Source: CAD feature listing. Evaluate the final solid. Frame: model axes, mm. A direction names the side the tool comes from. Give positions to 0.01 mm unless a question says otherwise; leave off trailing zeros. Order: outer loops, then holes, each group sorted by start corner. A loop starts at its lowest first (then second) coordinate and runs counter-clockwise, first axis right, second up. Notation, with made-up numbers: M 41.25,56 L 74.25,56 A32 cw 74.25,82 Z; hole C 67,-28.5 d9. An arc over 180 degrees is marked long. Return JSON: item names as keys, results as strings.
Autodesk Inventor part; units mm, degrees
ref_plane "YZ Plane" through (0, 0, 0) normal (1, 0, 0) x (0, 1, 0)
ref_plane "XZ Plane" through (0, 0, 0) normal (0, 1, 0) x (-1, 0, 0)
ref_plane "XY Plane" through (0, 0, 0) normal (0, 0, 1) x (1, 0, 0)
sketch "Sketch1" plane through (0, 0, 0) normal (0, 0, 1) x (1, 0, 0)
  line L0 (-84.0821, 192.7052) -> (642.9929, 192.7052)
  line L1 (642.9929, 192.7052) -> (642.9929, -137.4948)
  line L2 (642.9929, -137.4948) -> (-84.0821, -137.4948)
  line L3 (-84.0821, -137.4948) -> (-84.0821, 192.7052)
  circle A0 centre (131.8179, -91.7748) radius 25.4
  circle A1 centre (318.0537, 116.5052) radius 12.7
  line L4 (642.9929, -137.4948) -> (592.1929, -137.4948)
  line L5 (592.1929, -137.4948) -> (592.1929, -73.9948)
  line L6 (592.1929, -73.9948) -> (642.9929, -73.9948)
  line L7 (642.9929, -73.9948) -> (642.9929, -137.4948)
  line L8 (642.9929, 192.7052) -> (592.6352, 192.7052)
  line L9 (642.9929, 2.2052) -> (642.9929, 192.7052)
  line L10 (-84.0821, 53.0052) -> (5.7204, 53.0052) construction
  line L11 (-84.0821, 65.7052) -> (68.3179, -137.4948)
  line L12 (595.3679, 192.7052) -> (595.3679, 2.2052)
  line L13 (595.3679, 2.2052) -> (642.9929, 2.2052)
  point P0 (0, 0)
  dimension "d0" = 727.075
  dimension "d2" = 50.8
  dimension "d3" = 25.4
  dimension "d4" = 215.9
  dimension "d5" = 279.4
  dimension "d14" = 152.4
  dimension "d15" = 203.2
  dimension "d16" = 330.2
  dimension "d17" = 63.5
  dimension "d19" = 50.8
  dimension "d20" = 139.7
  dimension "d21" = 45.72
  dimension "d22" = 254
extrude "Extrusion1" add sketch "Sketch1" along normal blind 9.525 contours L0 L12 L13 L1 L6 L5 L2 L11 L3
sketch "Sketch3" plane through (0, 0, 9.525) normal (0, 0, 1) x (1, 0, 0)
  line L0 (595.3679, 2.2052) -> (595.3679, 192.7052)
  line L1 (595.3679, 192.7052) -> (-84.0821, 192.7052)
  line L2 (-84.0821, 192.7052) -> (-84.0821, 65.7052)
  line L3 (-84.0821, 127.1732) -> (106.4179, 192.7052)
  line L4 (595.3679, 2.2052) -> (684.2679, 2.2052)
  line L5 (684.2679, 2.2052) -> (684.2679, 40.3052)
  line L6 (684.2679, 40.3052) -> (595.3679, 40.3052)
  line L7 (595.3679, 40.3052) -> (595.3679, 2.2052)
  line L8 (684.2679, 40.3052) -> (379.4679, 192.7052)
  line L9 (595.3679, 40.3052) -> (595.3679, 84.7552)
  line L10 (595.3679, 84.7552) -> (595.3679, 192.7052)
  point P0 (0, 0)
  dimension "d32" = 190.5
  dimension "d33" = 65.532
  dimension "d38" = 88.9
  dimension "d39" = 38.1
  dimension "d40" = 215.9
extrude "Extrusion4" cut sketch "Sketch3" against normal blind 9.525 contours L3 L2 L1 | L8 L1 L0 | L0 L8 L6
sketch "Sketch4" plane through (0, 0, 9.525) normal (0, 0, 1) x (1, 0, 0)
  line L0 (595.3679, 2.2052) -> (595.3679, 84.7552)
  line L1 (595.3679, 84.7552) -> (379.4679, 192.7052)
  line L2 (595.3679, 84.7552) -> (684.2679, 40.3052)
  line L3 (684.2679, 40.3052) -> (595.3679, 40.3052)
  point P0 (0, 0)
  dimension "d43" = 88.9
extrude "Extrusion5" add sketch "Sketch4" against normal blind 9.525
sketch "Sketch5" plane through (0, 0, 9.525) normal (0, 0, 1) x (1, 0, 0)
  line L0 (642.9929, 2.2052) -> (592.1929, 2.2052)
  line L1 (592.1929, 2.2052) -> (592.1929, -73.9948)
  line L2 (592.1929, -73.9948) -> (642.9929, -73.9948)
  line L3 (642.9929, -73.9948) -> (642.9929, 2.2052)
  point P0 (0, 0)
extrude "Extrusion6" cut sketch "Sketch5" against normal blind 9.525
sketch "Sketch6" plane through (0, 0, 9.525) normal (0, 0, 1) x (1, 0, 0)
  line L0 (592.1929, -137.4948) -> (592.1929, 2.2052)
  line L1 (646.1679, 91.1052) -> (723.1394, 91.1052)
  line L2 (723.1394, 91.1052) -> (723.1394, -6.7385)
  line L3 (723.1394, -6.7385) -> (646.1679, -6.7385)
  line L4 (646.1679, -6.7385) -> (646.1679, 91.1052)
  line L5 (595.3679, 2.2052) -> (592.1929, 2.2052)
  line L6 (592.1929, 2.2052) -> (592.1929, 40.3052)
  line L7 (592.1929, 40.3052) -> (595.3679, 40.3052)
  line L8 (595.3679, 40.3052) -> (595.3679, 2.2052)
  point P0 (0, 0)
  dimension "d48" = 53.975
extrude "Extrusion7" cut sketch "Sketch6" against normal blind 9.525
sketch "Sketch8" plane through (0, 0, 9.525) normal (0, 0, 1) x (1, 0, 0)
  line L0 (-84.0821, 65.7052) -> (68.3179, -137.4948)
  line L1 (68.3179, -137.4948) -> (592.1929, -137.4948)
  line L2 (592.1929, -137.4948) -> (592.1929, 40.3052)
  line L3 (592.1929, -96.6594) -> (439.7929, -137.4948)
  line L4 (341.7489, -137.4948) -> (170.3104, -117.1748)
  line L5 (170.3104, -117.1748) -> (53.0779, -117.1748)
  point P0 (0, 0)
  dimension "d51" = 152.4
  dimension "d52" = 165
  dimension "d53" = 98.044
  dimension "d54" = 20.32
  dimension "d60" = 173.24
extrude "Extrusion8" cut sketch "Sketch8" against normal blind 9.525
sketch "Sketch9" plane through (0, 0, 9.525) normal (0, 0, 1) x (1, 0, 0)
  line L0 (592.1929, -96.6594) -> (592.1929, 40.3052)
  line L1 (646.1679, 40.3052) -> (592.1929, 40.3052)
  line L2 (592.1929, 40.3052) -> (592.1929, 5.3802)
  line L3 (592.1929, 5.3802) -> (646.1679, 5.3802)
  line L4 (646.1679, 5.3802) -> (646.1679, 40.3052)
  point P0 (0, 0)
  dimension "d57" = 34.925
extrude "Extrusion9" add sketch "Sketch9" against normal blind 9.525
sketch "Sketch10" plane through (0, 0, 9.525) normal (0, 0, 1) x (1, 0, 0)
  line L0 (-84.0821, 65.7052) -> (53.0779, -117.1748)
  line L1 (-84.0821, 127.1732) -> (-84.0821, 65.7052)
  line L2 (53.0779, -117.1748) -> (170.3104, -117.1748)
  arc A0 (82.3351, -98.9312) -> (-55.5071, 27.6052) centre (-44.6649, -98.9312) ccw
  line L3 (341.7489, -137.4948) -> (439.7929, -137.4948)
  line L4 (82.3351, -117.1748) -> (82.3351, -75.9981)
  point P0 (0, 0)
  point P1 (81.0179, -117.1748)
  point P2 (131.8179, -117.1748)
  dimension "d62" = 38.1
  dimension "d65" = 127
  dimension "d66" = 165.1
extrude "Extrusion10" cut sketch "Sketch10" against normal blind 25.4
sketch "Sketch12" plane through (0, 0, 9.525) normal (0, 0, 1) x (1, 0, 0)
  circle A0 centre (131.8179, -91.7748) radius 25.4
  circle A1 centre (131.8179, -91.7748) radius 38.1
  point P0 (0, 0)
  dimension "d70" = 76.2
extrude "Extrusion12" cut sketch "Sketch12" against normal blind 9.525
sketch "Sketch14" plane through (0, 0, 9.525) normal (0, 0, 1) x (1, 0, 0)
  arc A0 (160.2159, -117.1748) -> (103.4198, -117.1748) centre (131.8179, -91.7748) ccw
  line L0 (160.2159, -117.1748) -> (170.3104, -117.1748)
  line L1 (170.3104, -117.1748) -> (341.7489, -137.4948)
  line L2 (82.3351, -117.1748) -> (103.4198, -117.1748)
  circle A1 centre (131.8179, -91.7748) radius 38.1
  line L3 (341.7489, -137.4948) -> (82.3351, -137.4948)
  line L4 (82.3351, -137.4948) -> (82.3351, -117.1748)
  point P0 (0, 0)
  dimension "d74" = 20.32
extrude "Extrusion13" add sketch "Sketch14" against normal blind 9.525 contours L0 L1 L3 L4 L2 A1
sketch "Sketch15" plane through (0, 0, 9.525) normal (0, 0, 1) x (1, 0, 0)
  circle A0 centre (131.8179, -91.7748) radius 38.1
  line L0 (82.3351, -98.9312) -> (82.3351, -137.4948)
  line L1 (82.3351, -137.4948) -> (439.7929, -137.4948)
  circle A1 centre (185.7929, -51.1348) radius 76.2
  circle A2 centre (373.8763, -101.9348) radius 76.2
  line L2 (82.3351, -110.8248) -> (177.5851, -110.8248)
  line L3 (177.5851, -110.8248) -> (177.5851, -72.7248)
  line L4 (177.5851, -72.7248) -> (82.3351, -72.7248)
  line L5 (82.3351, -72.7248) -> (82.3351, -110.8248)
  line L6 (236.6324, -107.8955) -> (341.4074, -137.4948)
  line L7 (-84.0821, 127.1732) -> (-84.0821, 65.7052)
  line L8 (131.8179, -129.8748) -> (175.334, -129.8748)
  line L9 (131.8179, -129.8748) -> (82.3351, -129.8748)
  line L10 (236.6324, -107.8955) -> (142.6601, -129.8748)
  point P0 (0, 0)
  point P1 (154.0824, -137.4948)
  dimension "d77" = 152.4
  dimension "d78" = 53.975
  dimension "d79" = 40.64
  dimension "d80" = 152.4
  dimension "d81" = 291.5412
  dimension "d82" = 35.56
  dimension "d84" = 95.25
  dimension "d85" = 38.1
  dimension "d86" = 26.67
  dimension "d87" = 82.55
  dimension "d90" = 104.775
  dimension "d101" = 60.325
sketch "Sketch17" plane through (0, 0, 9.525) normal (0, 0, 1) x (1, 0, 0)
  line L0 (439.7929, -137.4948) -> (592.1929, -96.6594)
  line L1 (592.1929, -96.6594) -> (592.1929, 5.3802)
  line L2 (592.1929, -79.2096) -> (439.7929, -137.4948)
  point P0 (0, 0)
  dimension "d94" = 17.4498
extrude "Extrusion16" cut sketch "Sketch17" against normal blind 9.525
extrude "Extrusion18" cut sketch "Sketch15" against normal blind 9.525 contours L8 L10 A1 L6 A2 L1 L0 L9 | L10 A1 | L6 L1 A2 picked at (315.3812, -131.2856)
sketch "Sketch20" plane through (0, 0, 9.525) normal (0, 0, 1) x (1, 0, 0)
  circle A0 centre (131.8179, -91.7748) radius 38.1
  circle A1 centre (131.8179, -91.7748) radius 25.4
  point P0 (0, 0)
  dimension "d102" = 50.8
extrude "Extrusion19" add sketch "Sketch20" against normal blind 9.525
sketch "Sketch21" plane through (0, 0, 9.525) normal (0, 0, 1) x (1, 0, 0)
  line L0 (-84.0821, 65.7052) -> (-55.5071, 27.6052)
  arc A0 (82.3351, -98.9312) -> (-55.5071, 27.6052) centre (-44.6649, -98.9312) ccw
  line L1 (-84.0821, 65.7052) -> (-43.4592, 28.0631)
  point P0 (0, 0)
extrude "Extrusion20" cut sketch "Sketch21" against normal blind 9.525
properties part number "ShooterMountLeft_NERDS"
1. Set-up query: faces 1 (the face through (288.29, -122.49, 4.83)), 2 (the face through (510.951, 126.964, 4.829)). Return all of +Z, -Z, +X, -X, +Y, -Y with unobstructed straight access to the full face (end or side cutting, diameter ignored); none if empty.
Evaluation:
{"face 1": "+Z, -Z, -Y", "face 2": "+Z, -Z, +X, +Y"}
2. First-contact query: pin 1 (3 mm diameter, centred on y = -117, z = 6, fed in from -X); pin 2 (4 mm diameter, centred on y = -31, z = 8, fed in from +X); pin 3 (3 mm diameter, centred on x = 43.5, z = 4, fed in from +Y). Flat tips, straight axial feed; report the tip coordinate or a pass-through.
Evaluation:
{"pin 1": "stops at x = 82.34", "pin 2": "stops at x = 592.19", "pin 3": "stops at y = 171.58"}
3. Section query B-B (y = -53). Return loops of the section in (x, z) (3 decimals), then the cut area to 3 significant figures.
Evaluation:
{"outline": "M 73.738,0 L 592.193,0 L 592.193,9.525 L 73.738,9.525 Z", "area": "4,940 mm^2"}
4. Section query A-A (z = 5.5). Return loops of the section in (x, y), then the cut area to 3 significant figures.
Evaluation:
{"outline": "M -84.08,65.71 L -43.46,28.06 A127 cw 82.34,-98.93 L 82.34,-129.87 L 142.66,-129.87 L 236.63,-107.9 L 341.41,-137.49 L 439.79,-137.49 L 592.19,-79.21 L 592.19,5.38 L 646.17,5.38 L 646.17,59.36 L 379.47,192.71 L 106.42,192.71 L -84.08,127.17 Z; hole C 131.82,-91.77 d50.8; hole C 318.05,116.51 d25.4", "area": "174,000 mm^2"}
5. Draft query along X for faces 3 (the face through (330.167, 112.69, 4.696)), 4 (the face through (517.06, -107.944, 4.829)), 5 (the face through (276, 30, 9.525)), 6 (the face through (46.534, -10.547, 4.829)). Return one class per face: pulls with the +X half, pulls with the -X half, needs draft (parallel to the pull), parting line crosses it, or undercut.
Evaluation:
{"face 3": "undercut", "face 4": "pulls with the +X half", "face 5": "needs draft", "face 6": "pulls with the -X half"}
6. Ray query, probe 1 along Y at (x, z) = (317.5, 7.5); probe 2 along Y at (x, z) = (155, 1.5); probe 3 along Y at (x, z) = (275, 2.5). Return the intervals inside material, ascending.
Evaluation:
{"probe 1": "y = -130.74 to 103.82, 129.19 to 192.71", "probe 2": "y = -126.99 to -102.16, -81.39 to 192.71", "probe 3": "y = -118.73 to 192.71"}
7. Section query C-C (x = 223). Return loops of the section in (y, z) (3 decimals).
Evaluation:
{"outline": "M -111.084,0 L 192.705,0 L 192.705,9.525 L -111.084,9.525 Z"}
